Geometry: final body of the model. Coordinates: model frame, mm. Give positions to 0.01 mm unless a question says otherwise; leave off trailing zeros. Write each loop counter-clockwise with the first axis right and the second up, starting at its lowest first coordinate (ties: lowest second). Pieces come first, ordered by that corner, then holes. Notation, with made-up numbers: (-7.75, 64.5) -> (35.25, 64.5) arc R24 ccw to (35.25, 74.5) -> close; hole circle Ø1 at (-7.75, 42). An arc over 180 degrees is marked (long way). Answer in a Markdown table with one row per item. Add a question column.
Item 1: Material intervals for probe 1 along X at (y, z) = (-281.5, 14.5); probe 2 along X at (y, z) = (-215, 14.75); probe 3 along X at (y, z) = (-414, 10.5), sorted ascending. Write a range as from..to.
Item 2: Section query A-A on y = -25.4. Output: boundary loops of the cut face in (x, z), plus the area to 3 significant figures.
Item 3: First-contact query: P1, Ø1, axis at x = -71, z = 4.5, coming from the -Y side; P2, Ø1, axis at y = -73.5, z = 7.5, coming from the +X side; P3, Ø15, axis at x = -70.37, y = -432.83, coming from the -Z side. Flat tips, straight axial feed; report the tip coordinate or a pass-through.
Item 4: Section query B-B on x = -25.4. Output: boundary loops of the cut face in (y, z), plus the area to 3 significant figures.
Item 5: Section query D-D on y = -209.5. Output: boundary loops of the cut face in (x, z), plus the area to 3 significant figures.
Item 6: Section query C-C on z = 12. Output: boundary loops of the cut face in (x, y).
```python
from build123d import *

# Parameters (mm, degrees)
F0_W     = 50.8
F0_H     = 25.4
F1_DEPTH = 304.8
F3_DEPTH = 25.4
F4_R     = 12.7
F5_DEPTH = 25.4
F6_R     = 12.7
F7_DEPTH = 25.4
F8_R     = 12.7
F9_DEPTH = 25.4


with BuildPart() as f1:
    # F0 (on Front) → F1 (new body)
    with BuildSketch(Plane.XZ):
        with Locations((-25.4, 12.7)):
            Rectangle(F0_W, F0_H)
    extrude(amount=F1_DEPTH)

    # F2 (on face) → F3 (join)
    with BuildSketch(Plane.XY.offset(25.4)):
        Polygon((0, -304.8), (-50.8, -304.8), (-102.92387, -448.009155), (-55.187485, -465.383779), align=None)
    extrude(amount=-F3_DEPTH)

    # F4 (on face) → F5 (cut)
    with BuildSketch(Plane.XY.offset(25.4)):
        with Locations((-25.4, -25.4)):
            Circle(F4_R)
    extrude(amount=-F5_DEPTH, mode=Mode.SUBTRACT)

    # F6 (on face) → F7 (cut)
    with BuildSketch(Plane.XY.offset(25.4)):
        with Locations((-70.368366, -432.828274)):
            Circle(F6_R)
    extrude(amount=-F7_DEPTH, mode=Mode.SUBTRACT)

    # F8 (on face) → F9 (cut)
    with BuildSketch(Plane.XY.offset(25.4)):
        with Locations((-25.4, -280.161023)):
            Circle(F8_R)
    extrude(amount=-F9_DEPTH, mode=Mode.SUBTRACT)


solid = f1.part
```
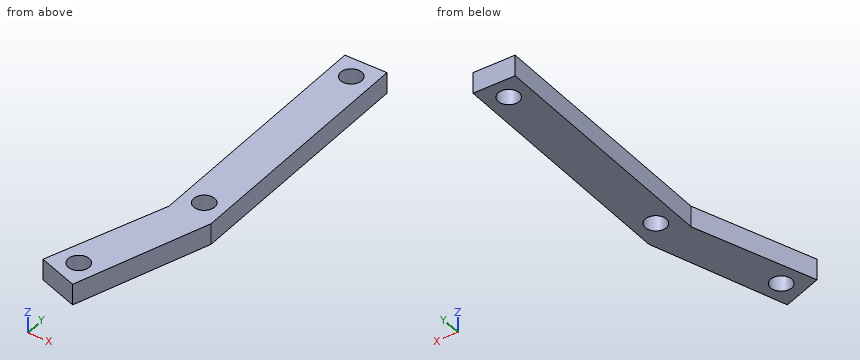
Findings below:
| question | item | result |
|---|---|---|
| 1 | probe 1 | x = -50.8..-38.03, -12.77..0 |
| 1 | probe 2 | x = -50.8..0 |
| 1 | probe 3 | x = -90.55..-37.53 |
| 2 | outline | (-50.8, 0) -> (-38.1, 0) -> (-38.1, 25.4) -> (-50.8, 25.4) -> close; (-12.7, 0) -> (0, 0) -> (0, 25.4) -> (-12.7, 25.4) -> close |
| 2 | area | 645 mm^2 |
| 3 | P1 | stops at y = -459.81 |
| 3 | P2 | stops at x = 0 |
| 3 | P3 | passes through |
| 4 | outline | (-378.71, 0) -> (-292.86, 0) -> (-292.86, 25.4) -> (-378.71, 25.4) -> close; (-267.46, 0) -> (-38.1, 0) -> (-38.1, 25.4) -> (-267.46, 25.4) -> close; (-12.7, 0) -> (0, 0) -> (0, 25.4) -> (-12.7, 25.4) -> close |
| 4 | area | 8,330 mm^2 |
| 5 | outline | (-50.8, 0) -> (0, 0) -> (0, 25.4) -> (-50.8, 25.4) -> close |
| 5 | area | 1,290 mm^2 |
| 6 | outline | (-102.92, -448.01) -> (-55.19, -465.38) -> (0, -304.8) -> (0, 0) -> (-50.8, 0) -> (-50.8, -304.8) -> close; hole circle Ø25.4 at (-70.37, -432.83); hole circle Ø25.4 at (-25.4, -280.16); hole circle Ø25.4 at (-25.4, -25.4) |
